Input: part model. Units: mm. Frame: model coordinates. Face numbers are marked on the shaded views. A direction names the side the tool comes from. Coordinates: 2 decimals unless noted, no trailing zeros. Order: outer loops, then holes, each group sorted by start corner. A loop starts at its lowest first (then second) coordinate and runs counter-clockwise, first axis right, second up. Notation, with made-up numbers: (30.5, 14) -> (65.5, 14) arc R16 cw to (65.5, 41) -> close; hole circle Ø10 at (20, -9.75). An arc over 180 degrees is marked (long way). Write each question's results on one line, items separated by ' | '.
```python
from build123d import *
from build123d.topology import SkipClean

# Parameters (mm, degrees)
CROQUIS2_R                 = 7.5
SALIENTE_EXTRUIR3_DEPTH    = 20
CROQUIS6_R                 = 30
SALIENTE_EXTRUIR4_DEPTH    = 25
CORTAR_EXTRUIR1_DEPTH      = 35
CORTAR_EXTRUIR1_DEPTH_BACK = 31
CROQUIS9_W                 = 20.718126327
CROQUIS9_H                 = 25
SALIENTE_EXTRUIR5_DEPTH    = 30
CORTAR_EXTRUIR2_DEPTH      = 15
CORTAR_EXTRUIR2_DEPTH_BACK = 38
CROQUIS11_R                = 5.492388524


with BuildPart() as part:
    # Croquis2 → Saliente-Extruir3 (new body)
    with BuildSketch(Plane(origin=(0, 0, 0), x_dir=(1, 0, 0), z_dir=(0, 1, 0))):
        with BuildLine():
            Line((-75, 15), (-6.126443354, 29.36778323))
            ThreePointArc((-6.126443354, 29.36778323), (0, 30), (6.126443354, 29.36778323))
            Line((6.126443354, 29.36778323), (75, 15))
            ThreePointArc((75, 15), (90, 0), (75, -15))
            Line((75, -15), (6.126443354, -29.36778323))
            ThreePointArc((6.126443354, -29.36778323), (0, -30), (-6.126443354, -29.36778323))
            Line((-6.126443354, -29.36778323), (-75, -15))
            ThreePointArc((-75, -15), (-90, 0), (-75, 15))
        make_face()
        with Locations(Location((-75, 0, 0), (0, 0, 270))):
            Circle(CROQUIS2_R, mode=Mode.SUBTRACT)
        with Locations(Location((75, 0, 0), (0, 0, 270))):
            Circle(CROQUIS2_R, mode=Mode.SUBTRACT)
    extrude(amount=SALIENTE_EXTRUIR3_DEPTH)

    # Croquis6 → Saliente-Extruir4 (add)
    with SkipClean():  # the faces are left unmerged after this step: merging them gives an invalid solid
        with BuildSketch(Plane(origin=(0, 20, 0), x_dir=(1, 0, 0), z_dir=(0, 1, 0))):
            with Locations(Location((0, 0, 0), (0, 0, 78.216463204))):
                Circle(CROQUIS6_R)
        extrude(amount=SALIENTE_EXTRUIR4_DEPTH)

    # Croquis9 → Cortar-Extruir1 (cut, two sides: drawn at the far end of the back side and taken through both)
    with SkipClean():  # the faces are left unmerged after this step: merging them gives an invalid solid
        with BuildSketch(Plane(origin=(0, 0, 0), x_dir=(0, 0, -1), z_dir=(1, 0, 0)).offset(-CORTAR_EXTRUIR1_DEPTH_BACK)):
            with Locations((0.502867144, 32.5)):
                Rectangle(CROQUIS9_W, CROQUIS9_H)
        extrude(amount=CORTAR_EXTRUIR1_DEPTH + CORTAR_EXTRUIR1_DEPTH_BACK, mode=Mode.SUBTRACT)

    # Croquis10 → Saliente-Extruir5 (add)
    with SkipClean():  # the faces are left unmerged after this step: merging them gives an invalid solid
        with BuildSketch(Plane(origin=(0, 45, 0), x_dir=(1, 0, 0), z_dir=(0, 1, 0))):
            Polygon((-24.500615631, 17.312418483), (24.500615631, 17.312418483), (27.964593149, 10.861930307), (-27.964593149, 10.861930307), align=None)
            Polygon((-28.334703105, -9.85619602), (-24.500615631, -17.312418483), (24.500615631, -17.312418483), (28.334703105, -9.85619602), align=None)
        extrude(amount=SALIENTE_EXTRUIR5_DEPTH)

    # Croquis11 → Cortar-Extruir2 (cut, two sides: drawn at the far end of the back side and taken through both)
    with SkipClean():  # the faces are left unmerged after this step: merging them gives an invalid solid
        with BuildSketch(Plane.XY.offset(17.312418483).offset(-CORTAR_EXTRUIR2_DEPTH_BACK)):
            with Locations(Location((0, 62.511511295, 0), (0, 0, 180))):
                Circle(CROQUIS11_R)
        extrude(amount=CORTAR_EXTRUIR2_DEPTH + CORTAR_EXTRUIR2_DEPTH_BACK, mode=Mode.SUBTRACT)


solid = part.part
```
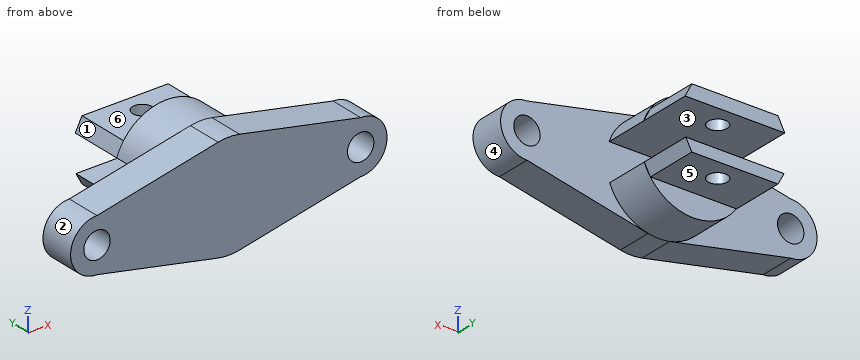
(1) Reachability of the marked faces 4, 5 and 6 from +Z, -Z, +X, -X, +Y, -Y: full face, straight path, thin tool, end or side. Return the list, or none.
Return value:
face 4: +X, +Y, -Y | face 5: -Z, +X, -X, +Y | face 6: +Z, +X, -X, +Y
(2) Cut plane B-B, the plane y = 51.5. Return loops of the section in (x, z), plus the area to 3 significant figures.
Return value:
outline: (-28.33, 9.86) -> (28.33, 9.86) -> (24.5, 17.31) -> (-24.5, 17.31) -> close; (-27.96, -10.86) -> (-24.5, -17.31) -> (24.5, -17.31) -> (27.96, -10.86) -> close | area: 732 mm2
(3) Mould query, pull axis Z, two halves, no side actions, for the marked faces 1, 2 and 3. Classes: +Z half, -Z half, draft (parallel to the pull), parting line (faces both ways), or undercut.
Return value:
face 1: +Z half | face 2: parting line | face 3: undercut
(4) Cut plane C-C, the plane x = 0. Return loops of the section in (y, z), plus the area to 3 significant figures.
Return value:
outline: (0, -30) -> (45, -30) -> (45, -17.31) -> (57.02, -17.31) -> (57.02, -10.86) -> (20, -10.86) -> (20, 9.86) -> (57.02, 9.86) -> (57.02, 17.31) -> (45, 17.31) -> (45, 30) -> (0, 30) -> close; (68, -17.31) -> (75, -17.31) -> (75, -10.86) -> (68, -10.86) -> close; (68, 9.86) -> (75, 9.86) -> (75, 17.31) -> (68, 17.31) -> close | area: 2,450 mm2
(5) Cut plane D-D, the plane y = 9. Return loops of the section in (x, z).
Return value:
outline: (-75, -15) -> (-6.13, -29.37) arc R30 ccw to (6.13, -29.37) -> (75, -15) arc R15 ccw to (75, 15) -> (6.13, 29.37) arc R30 ccw to (-6.13, 29.37) -> (-75, 15) arc R15 ccw to start; hole circle Ø15 at (-75, 0); hole circle Ø15 at (75, 0)
(6) Line query: line 1 along Y through (x, z) = (0, -15); line 2 along Y through (x, z) = (5, 27); line 3 along Y through (x, z) = (-61, 11.5). Output: solid intervals per line, ascending. Write a range as from..to.
Return value:
line 1: 0..57.02, 68..75 | line 2: 0..45 | line 3: 0..20
(7) Pin query (flat end, axial travel): P1, Ø3, axis at x = -49, z = -18, coming from the +Y side; P2, Ø15, axis at x = -9, y = 53.5, coming from the +Z side; P3, Ø4, axis at x = 5, z = -21, coming from the +Y side; P4, Ø12, axis at y = 32, z = -1, coming from the -X side. Return the tip coordinate at first contact, or that it passes through.
Return value:
P1: y = 20 | P2: z = 17.31 | P3: y = 45 | P4: through
(8) Cut plane A-A, the plane z = 0. Return loops of the section in (x, y), plus the area to 3 significant figures.
Return value:
outline: (-90, 0) -> (-82.5, 0) -> (-82.5, 20) -> (-90, 20) -> close; (-67.5, 0) -> (67.5, 0) -> (67.5, 20) -> (-67.5, 20) -> close; (82.5, 0) -> (90, 0) -> (90, 20) -> (82.5, 20) -> close | area: 3,000 mm2
